Part model, mm, in its own coordinate system. A direction names the side the tool comes from. Give positions to 0.01 mm unless a question says otherwise; leave off trailing zeros. Loops run counter-clockwise (first coordinate to the right, second up) from the corner with the lowest first, then second, coordinate; pieces in that order, holes last. Notation, with made-up numbers: (-1, -21) -> (13, -21) arc R20 ccw to (13, -15) -> close; hole circle Ø2 at (15.25, 12.5). An arc over 180 degrees is marked (long way). One line per question, with ' | ' between items.
```python
from build123d import *

# Parameters (mm, degrees)
F0_W     = 30
F0_H     = 35
F1_DEPTH = 10
F3_DEPTH = 10.001


# Not quite as in the source:
# - ends of sketch curves that miss each other by under 0.0002 mm in the source are joined


with BuildPart() as f1:
    # F0 (on Front) → F1 (new body)
    with BuildSketch(Plane.XZ):
        with Locations((15, 17.5)):
            Rectangle(F0_W, F0_H)
    extrude(amount=F1_DEPTH)

    # F2 (on face) → F3 (cut, through all)
    with BuildSketch(Plane.XZ.offset(10)):
        with BuildLine():
            Line((2.000000095, 7.3150651013), (2.000000095, 7))
            ThreePointArc((2.000000095, 7), (6.4219498037, 2.0335266063), (11.8663431882, 5.8516516319))
            ThreePointArc((11.8663431882, 5.8516516319), (13.0416655427, 8.0761900401), (15.1515475464, 9.4467197541))
            Line((15.1515475464, 9.4467197541), (19.1366200095, 10.7750772419))
            ThreePointArc((19.1366200095, 10.7750772419), (24.8292858299, 14.9607668958), (27.0000007004, 21.6849351694))
            Line((27.0000007004, 21.6849351694), (27.0000007004, 22))
            ThreePointArc((27.0000007004, 22), (22.5780501979, 26.9664733935), (17.1336568125, 23.1483483711))
            ThreePointArc((17.1336568125, 23.1483483711), (15.9583344576, 20.9238099649), (13.8484524551, 19.553280252))
            Line((13.8484524551, 19.553280252), (9.8633807858, 18.2249230289))
            ThreePointArc((9.8633807858, 18.2249230289), (4.1707149655, 14.0392333749), (2.000000095, 7.3150651013))
        make_face()
    extrude(amount=-F3_DEPTH, mode=Mode.SUBTRACT)


solid = f1.part
```
1) Saw through at C-C (x = 15.75). Give the cut face in (y, z), and give its area (3 significant figures).
Found:
outline: (-10, 0) -> (0, 0) -> (0, 9.65) -> (-10, 9.65) -> close; (-10, 20.71) -> (0, 20.71) -> (0, 35) -> (-10, 35) -> close | area: 239 mm2
2) Tool access for faces 4 (the cylindrical face through (4.23, -5.07, 14.12)), 5 (the flat face through (15, 0, 22)): list every direction of +Z, -Z, +X, -X, +Y, -Y with a clear straight run to the whole face (end or side of a thin tool).
Found:
face 4: +Y, -Y | face 5: +Z, -Z, +X, -X, +Y
3) Pin check, flat tip, straight feed: P1, Ø6, axis at x = 4, z = 9.5, coming from the +Y side. Stop position of the tip, or through.
Found:
P1: y = 0
4) Pull direction X, two halves, no side cores. Call faces 1 (the flat face through (0, -5, 17)), 2 (the flat face through (15, -5, 35)), 3 (the cylindrical face through (24.77, -5.07, 14.88)): pulls with the +X half, pulls with the -X half, needs draft (parallel to the pull), parting line crosses it, or undercut.
Found:
face 1: pulls with the -X half | face 2: needs draft | face 3: undercut
5) Saw through at A-A (y = -4.5). Give the cut face in (x, z), and give its area (3 significant figures).
Found:
outline: (0, 0) -> (30, 0) -> (30, 35) -> (0, 35) -> close; hole (2, 7) arc R5 ccw to (11.87, 5.85) arc R5 cw to (15.15, 9.45) -> (19.14, 10.78) arc R11.5 ccw to (27, 21.68) -> (27, 22) arc R5 ccw to (17.13, 23.15) arc R5 cw to (13.85, 19.55) -> (9.86, 18.22) arc R11.5 ccw to (2, 7.32) -> close | area: 735 mm2
6) Drill centre lines: line 1 (Z direction, x = 22.75, y = -2.25); line 2 (X direction, y = -0.5, z = 12); line 3 (Z direction, x = 16.5, y = -6.75). Where is each one in solid material? Low to high.
Found:
line 1: 0 to 12.76, 26.94 to 35 | line 2: 0 to 3, 21.7 to 30 | line 3: 0 to 9.9, 21.64 to 35
7) Saw through at B-B (z = 24.5). Give the cut face in (x, y), and give its area (3 significant figures).
Found:
outline: (0, -10) -> (17.67, -10) -> (17.67, 0) -> (0, 0) -> close; (26.33, -10) -> (30, -10) -> (30, 0) -> (26.33, 0) -> close | area: 213 mm2
